Check sheet for the drawn part. Datum: minimum x, y, z corner. Units: mm. Round coordinates to 2 decimals unless told otherwise and drop trailing zeros. Write each loop counter-clockwise with the first axis right and the second up, starting at its lowest first coordinate (ties: lowest second). Pieces come first, ordered by that corner, then holes. Notation, with made-up numbers: M 64.5,-34.5 L 115.5,-34.5 A9 cw 115.5,-24.5 Z; hole C 6.25,-39.75 d3. An arc over 180 degrees is marked long. Answer in a Markdown table with one row per item. Add a question column.
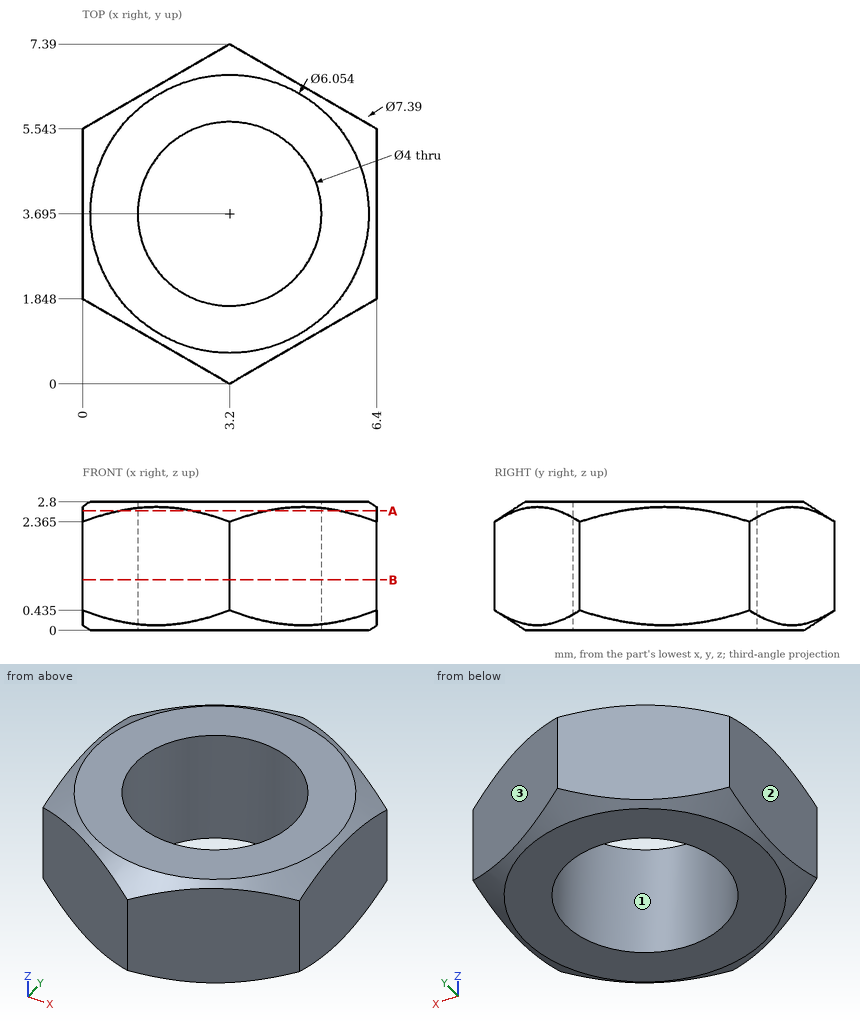
Item 1: Scan lines: probe 1 along Y at (x, z) = (3.5, 2.6) (1 decimal); probe 2 along X at (y, z) = (2.75, 0.55); probe 3 along Y at (x, z) = (3.25, 1.45) (1 decimal). Record each from-to range of solid material in increasing order. Write a range as from..to.
Item 2: Section check B-B, the plane z = 1.1. Record the boundary of the cut face in (x, y) (1 decimal), and give its area (3 significant figures).
Item 3: Mould release check, pull along X, two halves, no side actions. Record for the marked faces 1, 2 and 3: +X half, -X half, draft (parallel to the pull), parting line (faces both ways), or undercut.
Item 4: Section check A-A, the plane z = 2.6. Record the boundary of the cut face in (x, y) (1 decimal).
Item 5: Gauge pin test, flat end, axial feed: pin 1 Ø1 at (x, z) = (4.5, 0.5) entering from -Y. Record the tip position at first contact, or that the pin passes through.
Result sheet:
| question | item | result |
|---|---|---|
| 1 | probe 1 | y = 0.4..1.7, 5.7..7 |
| 1 | probe 2 | x = 0..1.44, 4.96..6.4 |
| 1 | probe 3 | y = 0..1.7, 5.7..7.4 |
| 2 | outline | M 0,1.8 L 3.2,0 L 6.4,1.8 L 6.4,5.5 L 3.2,7.4 L 0,5.5 Z; hole C 3.2,3.7 d4 |
| 2 | area | 22.9 mm^2 |
| 3 | face 1 | undercut |
| 3 | face 2 | -X half |
| 3 | face 3 | +X half |
| 4 | outline | M 0,2.8 A3.3 ccw 0.8,1.4 L 2.4,0.5 A3.3 ccw 4,0.5 L 5.6,1.4 A3.3 ccw 6.4,2.8 L 6.4,4.6 A3.3 ccw 5.6,6 L 4,6.9 A3.3 ccw 2.4,6.9 L 0.8,6 A3.3 ccw 0,4.6 Z; hole C 3.2,3.7 d4 |
| 5 | pin 1 | stops at y = 0.46 |
